```python
from build123d import *

# Parameters (mm, degrees)
ESQUISSE1_R        = 2.5
BOSS_EXTRU_1_DEPTH = 4


with BuildPart() as part:
    # Esquisse1 → Boss.-Extru.1 (new body)
    with BuildSketch(Plane.XY):
        Polygon((-5, -2.071067812), (-3.535533906, -3.535533906), (-2.071067812, -5), (2.071067812, -5), (3.535533906, -3.535533906), (5, -2.071067812), (5, 2.071067812), (3.535533906, 3.535533906), (2.071067812, 5), (-2.071067812, 5), (-3.535533906, 3.535533906), (-5, 2.071067812), (-5, 0), align=None)
        Circle(ESQUISSE1_R, mode=Mode.SUBTRACT)
    extrude(amount=BOSS_EXTRU_1_DEPTH)


solid = part.part
```
Check sheet for the modelled part. Datum: model origin and axes. Units: mm. Round coordinates to 2 decimals unless told otherwise and drop trailing zeros. Loops run counter-clockwise (first coordinate to the right, second up) from the corner with the lowest first, then second, coordinate; pieces in that order, holes last. Notation, with made-up numbers: M 22.25,85 L 63.25,85 A32 ccw 63.25,121 Z; hole C 8,40 d2. An arc over 180 degrees is marked long. Answer as a JSON object with one key per item and string values.
1. Mould release check, pull along X, two halves, no side actions. Record for faces 1 (the flat face through (0, 5, 2)), 2 (the flat face through (-3.515, 3.556, 1.972)), 3 (the cylindrical face through (-0.54, -2.44, 1.97)): pulls with the +X half, pulls with the -X half, needs draft (parallel to the pull), parting line crosses it, or undercut.
Reply:
{"face 1": "needs draft", "face 2": "pulls with the -X half", "face 3": "undercut"}
2. Scan lines: line 1 (Y direction, x = 0, z = 0.8); line 2 (Y direction, x = -1, z = 0.2); line 3 (X direction, y = 1.75, z = 2). Record each from-to range of solid material in increasing order.
Reply:
{"line 1": "y = -5 to -2.5, 2.5 to 5", "line 2": "y = -5 to -2.29, 2.29 to 5", "line 3": "x = -5 to -1.79, 1.79 to 5"}
3. Section check C-C (z = 1.6). Record the boundary of the cut face in (x, y), plus the area to 3 significant figures.
Reply:
{"outline": "M -5,-2.07 L -2.07,-5 L 2.07,-5 L 5,-2.07 L 5,2.07 L 2.07,5 L -2.07,5 L -5,2.07 Z; hole C 0,0 d5", "area": "63.2 mm²"}
4. Section check D-D (y = 3.5). Record the boundary of the cut face in (x, z), plus the area to 3 significant figures.
Reply:
{"outline": "M -3.57,0 L 3.57,0 L 3.57,4 L -3.57,4 Z", "area": "28.6 mm²"}
5. Section check A-A (x = 0). Record the boundary of the cut face in (y, z).
Reply:
{"outline": "M -5,0 L -2.5,0 L -2.5,4 L -5,4 Z; M 2.5,0 L 5,0 L 5,4 L 2.5,4 Z"}
6. Gauge pin test, flat end, axial feed: P1, Ø2, axis at x = 3.5, z = 0.5, coming from the -Y side. Record the tip position at first contact, or that the pin passes through.
Reply:
{"P1": "stops at y = -4.57"}
